from build123d import *

# Parameters (mm, degrees)
HOLE_WIZARD_1_D           = 6.6
HOLE_WIZARD_1_CSINK_D     = 12.8
HOLE_WIZARD_1_CSINK_ANGLE = 90
SKETCH_3_W                = 2
SKETCH_3_H                = 2.5
CUT_EXTRUDE_1_DEPTH       = 13.5
CUT_EXTRUDE_1_DEPTH_BACK  = 13.5


with BuildPart() as part:
    # 草图1 → 旋转1 (revolve)
    with BuildSketch(Plane.XY):
        Polygon((0, 0), (9.5, 0), (9.5, 5), (12.5, 5), (12.5, 7.5), (0, 7.5), align=None)
    revolve(axis=Axis((0, 11.114035088, 0), (0, -1, 0)))

    # 打孔尺寸(%根据)内六角花形半沉头螺钉的类型1 (through all)
    with Locations(Plane.ZX.offset(7.5)):
        with Locations((0, 0)):
            CounterSinkHole(HOLE_WIZARD_1_D / 2, HOLE_WIZARD_1_CSINK_D / 2, counter_sink_angle=HOLE_WIZARD_1_CSINK_ANGLE)

    # 草图3 → 切除-拉伸1 (cut, two sides)
    with BuildSketch(Plane.XY) as cut_extrude_1_sk:
        with Locations((-11.5, 6.25)):
            Rectangle(SKETCH_3_W, SKETCH_3_H)
        with Locations((11.5, 6.25)):
            Rectangle(SKETCH_3_W, SKETCH_3_H)
    extrude(amount=CUT_EXTRUDE_1_DEPTH, mode=Mode.SUBTRACT)
    extrude(cut_extrude_1_sk.sketch, amount=-CUT_EXTRUDE_1_DEPTH_BACK, mode=Mode.SUBTRACT)


solid = part.part
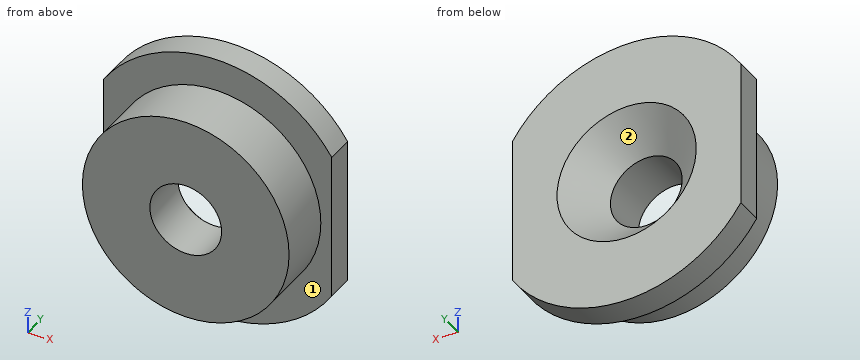
Input: part model. Units: mm. Frame: model coordinates. Face numbers are marked on the shaded views. A direction names the side the tool comes from. Coordinates: 2 decimals unless noted, no trailing zeros. Order: outer loops, then holes, each group sorted by start corner. A loop starts at its lowest first (then second) coordinate and runs counter-clockwise, first axis right, second up. Notation, with made-up numbers: M 33,43.25 L 50,43.25 A22 ccw 50,72.25 Z; hole C -9.75,31.5 d4. An arc over 180 degrees is marked long. Write item = value, one per line. Start each with the question number.
(1) Section C-C on y = 7. Output: boundary loops of the cut face in (x, z), and give its area (3 significant figures).
(2) Section A-A on x = 0. Output: boundary loops of the cut face in (y, z), and give its area (3 significant figures).
(3) Section B-B on z = 0. Output: boundary loops of the cut face in (x, y), and give its area (3 significant figures).
(4) Line query: line 1 along Z through (x, y) = (0, 1.6); line 2 along Y through (x, z) = (5.25, -8); line 3 along X through (y, z) = (1.25, 0.25). Output: solid intervals per line, ascending. Write a range as [from, to].
(5) Reachability of the marked faces 1 and 2 from +Z, -Z, +X, -X, +Y, -Y: full face, straight path, thin tool, end or side. Return the list, or none.
(6) First-contact query: P1, Ø3, axis at y = 4.5, z = -10, coming from the +X side; P2, Ø2, axis at y = 1.5, z = 7, coming from the +X side; P3, Ø5.5, axis at x = 0, z = 0, coming from the +Y side. Flat tips, straight axial feed; report the tip coordinate or a pass-through.
(7) Section D-D on x = 7.5. Output: boundary loops of the cut face in (y, z), and give its area (3 significant figures).
Result set:
q1.outline = M -10.5,-6.78 A12.5 ccw 10.5,-6.78 L 10.5,6.78 A12.5 ccw -10.5,6.78 Z; hole C 0,0 d11.8
q1.area = 345 mm²
q2.outline = M 0,-9.5 L 5,-9.5 L 5,-12.5 L 7.5,-12.5 L 7.5,-6.4 L 4.4,-3.3 L 0,-3.3 Z; M 0,3.3 L 4.4,3.3 L 7.5,6.4 L 7.5,12.5 L 5,12.5 L 5,9.5 L 0,9.5 Z
q2.area = 98.4 mm²
q3.outline = M -10.5,5 L -9.5,5 L -9.5,0 L -3.3,0 L -3.3,4.4 L -6.4,7.5 L -10.5,7.5 Z; M 3.3,0 L 9.5,0 L 9.5,5 L 10.5,5 L 10.5,7.5 L 6.4,7.5 L 3.3,4.4 Z
q3.area = 88.4 mm²
q4.line_1 = [-9.5, -3.3], [3.3, 9.5]
q4.line_2 = [5, 7.5]
q4.line_3 = [-9.5, -3.29], [3.29, 9.5]
q5.face_1 = -Y
q5.face_2 = +Y
q6.P1 = 9.08
q6.P2 = 7.37
q6.P3 = through
q7.outline = M 0,-5.83 L 5,-5.83 L 5,-10 L 7.5,-10 L 7.5,10 L 5,10 L 5,5.83 L 0,5.83 Z
q7.area = 108 mm²
